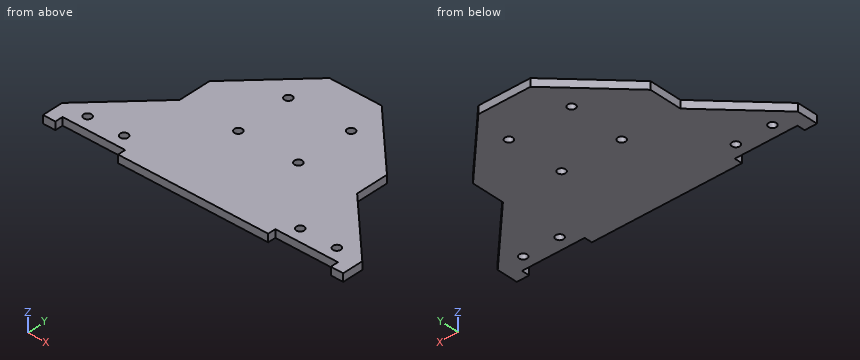
Autodesk Inventor part; units mm, degrees
ref_plane "YZ Plane" through (0, 0, 0) normal (1, 0, 0) x (0, 1, 0)
ref_plane "XZ Plane" through (0, 0, 0) normal (0, 1, 0) x (-1, 0, 0)
ref_plane "XY Plane" through (0, 0, 0) normal (0, 0, 1) x (1, 0, 0)
sketch "Эскиз1" plane through (0, 0, 0) normal (0, 0, 1) x (1, 0, 0)
  line L0 (57.5, -31.5) -> (-57.5, -31.5)
  line L1 (-57.5, -31.5) -> (-57.5, 31.5)
  line L2 (-57.5, 31.5) -> (57.5, 31.5)
  line L3 (57.5, 31.5) -> (57.5, -31.5)
  line L4 (57.5, -31.5) -> (-57.5, 31.5) construction
  line L5 (-57.5, -31.5) -> (57.5, 31.5) construction
  line L6 (0, 0) -> (0, 31.5)
  line L7 (0, 31.5) -> (12, 31.5)
  line L8 (12, 31.5) -> (12, 21.5)
  line L9 (12, 21.5) -> (0, 21.5)
  line L10 (0, 21.5) -> (0, 31.5)
  line L11 (0, 31.5) -> (-12, 31.5)
  line L12 (-12, 31.5) -> (-12, 21.5)
  line L13 (-12, 21.5) -> (0, 21.5)
  line L14 (0, 21.5) -> (0, 31.5)
  circle A0 centre (-12, 21.5) radius 1.5
  circle A1 centre (12, 21.5) radius 1.5
  line L15 (0, 0) -> (-33.75, 0)
  line L16 (-33.75, 0) -> (-33.75, -31.5)
  line L17 (-33.75, -31.5) -> (0, -31.5)
  line L18 (0, -31.5) -> (0, 0)
  line L19 (0, -31.5) -> (-33.75, -31.5)
  line L20 (-33.75, -31.5) -> (-33.75, -23.5)
  line L21 (-33.75, -23.5) -> (0, -23.5)
  line L22 (0, -23.5) -> (0, -31.5)
  line L23 (-57.5, -31.5) -> (57.5, -31.5)
  line L24 (57.5, -31.5) -> (57.5, -28.5)
  line L25 (57.5, -28.5) -> (-57.5, -28.5)
  line L26 (-57.5, -28.5) -> (-57.5, -31.5)
  circle A2 centre (-33.75, -23.5) radius 1.5
  line L27 (-33.75, -23.5) -> (-47.75, -23.5)
  line L28 (-47.75, -23.5) -> (-47.75, -31.5)
  line L29 (-47.75, -31.5) -> (-33.75, -31.5)
  line L30 (-33.75, -31.5) -> (-33.75, -23.5)
  circle A3 centre (-47.75, -23.5) radius 1.5
  line L31 (33.75, -31.5) -> (33.75, -23.5)
  circle A4 centre (33.75, -23.5) radius 1.5
  line L32 (47.75, -23.5) -> (47.75, -31.5)
  circle A5 centre (47.75, -23.5) radius 1.5
  line L33 (0, 0) -> (11.5, 0)
  circle A6 centre (11.5, 0) radius 1.5
  circle A7 centre (-11.5, 0) radius 1.5
  line L34 (-33.75, -31.5) -> (-28.75, -31.5)
  line L35 (-28.75, -31.5) -> (-28.75, -28.5)
  line L36 (-28.75, -28.5) -> (-33.75, -28.5)
  line L37 (-33.75, -28.5) -> (-33.75, -31.5)
  line L38 (-47.75, -31.5) -> (-52.75, -31.5)
  line L39 (-52.75, -31.5) -> (-52.75, -28.5)
  line L40 (-52.75, -28.5) -> (-47.75, -28.5)
  line L41 (-47.75, -28.5) -> (-47.75, -31.5)
  line L42 (28.75, -31.5) -> (28.75, -28.5)
  line L43 (52.75, -31.5) -> (52.75, -28.5)
  line L44 (-47.75, -23.5) -> (-57.5, -23.5)
  line L45 (-57.5, -23.5) -> (-34, 0)
  line L46 (-57.5, -23.5) -> (-24.266, -23.5) construction
  line L47 (-12, 31.5) -> (-34, 9.5)
  line L48 (-12, 31.5) -> (19.1127, 31.5) construction
  line L49 (-34, 9.5) -> (-34, 0)
  line L50 (-57.5, -31.5) -> (57.5, 31.5) construction
  line L51 (57.5, -23.5) -> (34, 0)
  line L52 (12, 31.5) -> (34, 9.5)
  line L53 (34, 9.5) -> (34, 0)
  line L54 (34, 9.5) -> (34, 31.5)
  line L55 (-34, 9.5) -> (-34, 31.5)
  line L56 (12, 31.5) -> (15, 31.5)
  line L57 (15, 31.5) -> (34, 12.5)
  line L58 (-12, 31.5) -> (-15, 31.5)
  line L59 (-15, 31.5) -> (-34, 12.5)
  line L60 (-57.5, 31.5) -> (57.5, 31.5)
  line L61 (57.5, 31.5) -> (57.5, 36.5)
  line L62 (57.5, 36.5) -> (-57.5, 36.5)
  line L63 (-57.5, 36.5) -> (-57.5, 31.5)
  line L64 (-15, 31.5) -> (-10, 36.5)
  line L65 (15, 31.5) -> (10, 36.5)
  point P0 (-47.75, -28.5)
  point P1 (-33.75, -28.5)
  point P2 (33.75, -28.5)
  point P3 (47.75, -28.5)
  dimension "d0" = 115
  dimension "d1" = 63
  dimension "d2" = 12
  dimension "d3" = 10
  dimension "d4" = 12
  dimension "d5" = 3
  dimension "d6" = 3
  dimension "d7" = 33.75
  dimension "d8" = 8
  dimension "d9" = 3
  dimension "d10" = 3
  dimension "d11" = 14
  dimension "d12" = 3
  dimension "d13" = 11.5
  dimension "d14" = 3
  dimension "d17" = 5
  dimension "d18" = 5
  dimension "d19" = 45
  dimension "d20" = 135
  dimension "d21" = 3
  dimension "d22" = 135
  dimension "d23" = 3
  dimension "d24" = 5
extrude "Выдавливание1" add sketch "Эскиз1" along normal blind 3 contours L0 L43 L25 L3 | L25 L18 L6 L9 A1 L8 L52 L53 L51 L3 | L0 L18 L25 L42 | L52 L2 L57 L54 | L0 L35 L25 L18 | L2 L64 L62 L65 | L8 A1 L9 L6 L2 | L25 L16 A2 L21 L18 | L6 L13 A0 L12 L2 | L21 A2 L16 L15 A7 L18 | L2 L47 L55 L59 | L12 A0 L13 L6 L15 A7 L16 A2 L27 A3 L44 L45 L49 L47 | L25 L28 A3 L27 A2 L16 | L0 L1 L25 L39 | L25 L1 L44 A3 L28
properties part number "дно"
The listing builds one solid part. Answer for the finished solid, in the listing's coordinates (mm). Give positions to 0.01 mm unless a question says otherwise; leave off trailing zeros. Loops run counter-clockwise (first coordinate to the right, second up) from the corner with the lowest first, then second, coordinate; pieces in that order, holes last. Notation, with made-up numbers: (27.5, 24.25) - (57.5, 24.25) arc R16 cw to (57.5, 28.25) - close; hole circle Ø3 at (-13.5, 46). An arc over 180 degrees is marked (long way). Use one line per item in the form item = value.
1. Find the intervals of material crossed by line 1 along X through (y, z) = (-23.5, 1.75); line 2 along X through (y, z) = (0, 0.95); line 3 along X through (y, z) = (21.5, 2.45), in increasing order. Write a range as [from, to].
Calculated:
line_1 = [-57.5, -49.25], [-46.25, -35.25], [-32.25, 32.25], [35.25, 46.25], [49.25, 57.5]
line_2 = [-34, -13], [-10, 10], [13, 34]
line_3 = [-25, -13.5], [-10.5, 10.5], [13.5, 25]
2. Section B-B on x = -24.5 is taken. Give the vertices of the cut face in (y, z), then the cut area to 4 significant figures.
Calculated:
outline = (-31.5, 0) - (22, 0) - (22, 3) - (-31.5, 3) - close
area = 160.5 mm^2
3. Section C-C on y = -9 is taken. Give the vertices of the cut face in (x, z), then the cut area to 3 significant figures.
Calculated:
outline = (-43, 0) - (43, 0) - (43, 3) - (-43, 3) - close
area = 258 mm^2
4. Section A-A on z = 0.8 is taken. Count the separate pieces of the cut face and the enclosed holes in it, then the cut area to 3 significant figures.
Calculated:
separate_pieces = 1
enclosed_holes = 8
area = 4,780 mm^2
5. Given pin 1 Ø2.5 at (x, y) = (33.75, -23.5) entering from +Z; pin 2 Ø1 at (x, z) = (38, 0.5) entering from +Y; pin 3 Ø1 at (x, z) = (41.5, 0.5) entering from +Y; pin 4 Ø1.5 at (x, z) = (44.5, 1.5) entering from -Y, each flat-ended and moving along its own axis, determine where each tip first touches the part or whether it passes through.
Calculated:
pin_1 = through
pin_2 = -3.5
pin_3 = -7
pin_4 = -28.5
